from build123d import *

# Parameters (mm, degrees)
SKETCH1_W           = 22.225
SKETCH1_H           = 63.5
SKETCH1_R           = 1.5875
BOSS_EXTRUDE1_DEPTH = 18.415
SKETCH2_R           = 6.985
BOSS_EXTRUDE2_DEPTH = 4.699
SKETCH3_R           = 31.75
BOSS_EXTRUDE3_DEPTH = 26.924


with BuildPart() as part:
    # Sketch1 → Boss-Extrude1 (new body)
    with BuildSketch(Plane.XY):
        with Locations((-21.669088448, 0.687725632)):
            Rectangle(SKETCH1_W, SKETCH1_H)
        with Locations((-30.368588448, 0.687725632)):
            Circle(SKETCH1_R, mode=Mode.SUBTRACT)
        with Locations((-12.969588448, 0.687725632)):
            Circle(SKETCH1_R, mode=Mode.SUBTRACT)
    extrude(amount=BOSS_EXTRUDE1_DEPTH)

    # Sketch2 → Boss-Extrude2 (add)
    with BuildSketch(Plane.XY.offset(18.415)):
        with Locations((-21.669088448, -21.918274368)):
            Circle(SKETCH2_R)
    extrude(amount=BOSS_EXTRUDE2_DEPTH)

    # Sketch3 → Boss-Extrude3 (add)
    with BuildSketch(Plane.XY.offset(23.114)):
        with Locations((-21.669088448, -21.918274368)):
            Circle(SKETCH3_R)
    extrude(amount=BOSS_EXTRUDE3_DEPTH)


solid = part.part
Design review of the part built by this model. Coordinates are the model's own, in mm. A direction names the side the tool comes from. Give positions to 0.01 mm unless a question says otherwise; leave off trailing zeros. Order: outer loops, then holes, each group sorted by start corner. A loop starts at its lowest first (then second) coordinate and runs counter-clockwise, first axis right, second up.
1. Tool access review of faces 4 (the cylindrical face through (-31.955, 0.758, 9.079)), 5 (the flat face through (-22, -31.062, 9)), 6 (the flat face through (-32.782, 0, 9)), 7 (the flat face through (-10.557, 0, 9)): name each direction out of +Z, -Z, +X, -X, +Y, -Y from which nothing blocks a thin tool from reaching the whole face with its end or side.
Solution:
face 4: -Z
face 5: -Z, +X, -X, -Y
face 6: -Z, -X, +Y, -Y
face 7: -Z, +X, +Y, -Y
2. Add section A-A, the plane y = 5.5. State the section outline as (x, z) points (3 decimals), then the cut area to 3 significant figures.
Solution:
outline: (-37.678, 23.114) - (-5.66, 23.114) - (-5.66, 50.038) - (-37.678, 50.038) - close; (-32.782, 0) - (-10.557, 0) - (-10.557, 18.415) - (-32.782, 18.415) - close
area: 1,270 mm2
3. Add section D-D, the plane y = -16. State the section outline as (x, z) points (3 decimals).
Solution:
outline: (-52.863, 23.114) - (-25.379, 23.114) - (-25.379, 18.415) - (-32.782, 18.415) - (-32.782, 0) - (-10.557, 0) - (-10.557, 18.415) - (-17.959, 18.415) - (-17.959, 23.114) - (9.524, 23.114) - (9.524, 50.038) - (-52.863, 50.038) - close
4. Add section B-B, the plane z = 7. State the section outline as (x, y) points (1 decimal).
Solution:
outline: (-32.8, -31.1) - (-10.6, -31.1) - (-10.6, 32.4) - (-32.8, 32.4) - close; hole circle Ø3.2 at (-30.4, 0.7); hole circle Ø3.2 at (-13, 0.7)
5. To check wall thickness, follow L1, parallel to X at y = -21, z = 44; L2, parallel to Z at x = -37, y = -14.5; L3, parallel to X at y = 24, z = 2. State the ranges of each line that lie inside material, in increasing order.
Solution:
L1: x = -53.41 to 10.07
L2: z = 23.11 to 50.04
L3: x = -32.78 to -10.56
6. Add section C-C, the plane x = -23.5. State the section outline as (y, z) points (1 decimal), then the cut area to 3 significant figures.
Solution:
outline: (-53.6, 23.1) - (-28.7, 23.1) - (-28.7, 18.4) - (-31.1, 18.4) - (-31.1, 0) - (32.4, 0) - (32.4, 18.4) - (-15.2, 18.4) - (-15.2, 23.1) - (9.8, 23.1) - (9.8, 50) - (-53.6, 50) - close
area: 2,940 mm2
7. For pin 1 Ø2 at (y, z) = (-14.5, 37.5) entering from -X; pin 2 Ø8 at (y, z) = (-32, 13) entering from +X; pin 3 Ø12 at (x, y) = (-0.5, -41.5) entering from -Z, all flat-tipped, find the tip position at first contact; note any pin that passes through.
Solution:
pin 1: stops at x = -52.76
pin 2: stops at x = -10.56
pin 3: stops at z = 23.11
8. Mouldability with a two-part tool opening along Y and no side actions: class faces 1 (the flat face through (-22, -21, 50.038)), 2 (the cylindrical face through (-11.503, 0.08, 9.079)), 3 (the cylindrical face through (-27.21, -26.17, 20.73)) as +Y half, -Y half, draft (parallel to the pull), parting line (faces both ways), or undercut.
Solution:
face 1: draft
face 2: undercut
face 3: parting line
